Autodesk Inventor part; units mm, degrees
ref_plane "YZ Plane" through (0, 0, 0) normal (1, 0, 0) x (0, 1, 0)
ref_plane "XZ Plane" through (0, 0, 0) normal (0, 1, 0) x (-1, 0, 0)
ref_plane "XY Plane" through (0, 0, 0) normal (0, 0, 1) x (1, 0, 0)
sketch "Sketch1" plane through (0, 0, 0) normal (0, 1, 0) x (-1, 0, 0)
  line L0 (0, -471.17) -> (0, 471.17)
  line L1 (1409.065, 0) -> (-1409.065, 0)
  line L2 (-1003.3, 333.375) -> (1003.3, 333.375)
  line L3 (1003.3, 333.375) -> (1003.3, -333.375)
  line L4 (1003.3, -333.375) -> (-1003.3, -333.375)
  line L5 (-1003.3, -333.375) -> (-1003.3, 333.375)
  line L6 (-968.375, 298.45) -> (968.375, 298.45)
  line L7 (968.375, 298.45) -> (968.375, -298.45)
  line L8 (968.375, -298.45) -> (-968.375, -298.45)
  line L9 (-968.375, -298.45) -> (-968.375, 298.45)
  line L10 (-1006.475, 336.55) -> (1006.475, 336.55)
  line L11 (1006.475, 336.55) -> (1006.475, -336.55)
  line L12 (1006.475, -336.55) -> (-1006.475, -336.55)
  line L13 (-1006.475, -336.55) -> (-1006.475, 336.55)
  point P0 (0, 0)
  dimension "d0" = 2006.6
  dimension "d1" = 666.75
  dimension "d2" = 596.9
  dimension "d3" = 1936.75
  dimension "d4" = 3.175
  dimension "d5" = 3.175
extrude "Extrusion1" add sketch "Sketch1" against normal blind 3.175 contours L12 L13 L1 L5 L4 L0 | L0 L4 L3 L1 L11 L12 | L4 L5 L1 L9 L8 L0 | L0 L8 L7 L1 L3 L4 | L1 L3 L2 L0 L10 L11 | L13 L10 L0 L2 L5 L1 | L1 L7 L6 L0 L2 L3 | L5 L2 L0 L6 L9 L1
extrude "Extrusion2" add sketch "Sketch1" along normal blind 34.925 contours L12 L13 L1 L5 L4 L0 | L0 L4 L3 L1 L11 L12 | L1 L3 L2 L0 L10 L11 | L13 L10 L0 L2 L5 L1
sketch "Sketch2" plane through (0, 34.925, 0) normal (0, 1, 0) x (1, 0, 0)
  line L0 (1006.475, -336.55) -> (1006.475, 336.55)
  line L1 (1006.475, 336.55) -> (-1006.475, 336.55)
  line L2 (971.55, 336.55) -> (1006.475, 336.55)
  line L3 (1006.475, 339.725) -> (971.55, 339.725)
  line L4 (971.55, 339.725) -> (971.55, 336.55)
  line L5 (1006.475, 339.725) -> (1009.65, 339.725)
  line L6 (1009.65, 339.725) -> (1009.65, 301.625)
  line L7 (1009.65, 301.625) -> (1006.475, 301.625)
  line L8 (1006.475, 301.625) -> (1006.475, 336.55)
  point P0 (0, 0)
  dimension "d10" = 3.175
  dimension "d15" = 3.175
  dimension "d41" = 38.1
  dimension "d42" = 38.1
extrude "Extrusion3" add sketch "Sketch2" against normal blind 381
sketch "Sketch4" plane through (1006.475, -3.175, 336.55) normal (1, 0, 0) x (0, 0, -1)
  line L0 (638.175, 0) -> (0, 0)
  line L1 (447.479, 24.9105) -> (420.7746, -2.2646)
  line L2 (420.7746, -2.2646) -> (638.175, -215.9)
  line L3 (638.175, -215.9) -> (638.175, -162.483)
  line L4 (638.175, -162.483) -> (447.479, 24.9105)
  line L5 (638.175, 38.1) -> (638.175, -342.9)
  line L6 (676.275, -342.9) -> (638.175, -342.9)
  line L7 (422.9999, 0) -> (638.175, -211.4486)
  line L8 (422.9999, 0) -> (420.7746, -2.2646)
  line L9 (420.7746, -2.2646) -> (638.175, -215.9)
  line L10 (638.175, -215.9) -> (638.175, -211.4486)
  line L11 (638.175, -211.4486) -> (422.9999, 0)
  point P0 (336.55, 3.175)
  dimension "d23" = 38.1
  dimension "d24" = 304.8
  dimension "d25" = 127
  dimension "d28" = 3.175
extrude "Extrusion5" add sketch "Sketch4" against normal blind 34.925 contours L7 L3 L2 L1
extrude "Extrusion6" add sketch "Sketch4" along normal blind 3.175 contours L4 L3 L7 L0 | L0 L1 L4 | L7 L3 L2 L1
sketch "Sketch5" plane through (1009.65, 34.925, -339.725) normal (0, 0, -1) x (-1, 0, 0)
  line L0 (38.1, -381) -> (0, -381)
  line L1 (38.1, 0) -> (38.1, -381)
  line L2 (38.1, 0) -> (38.1, -38.1)
  line L3 (2016.125, -38.1) -> (38.1, -38.1)
  line L4 (2016.125, 0) -> (2016.125, -38.1)
  line L5 (38.1, 0) -> (2016.125, 0)
  line L6 (38.1, -355.6) -> (369.2808, -40.3999)
  line L7 (369.2808, -40.3999) -> (343.0141, -12.8015)
  line L8 (343.0141, -12.8015) -> (38.1, -303.0024)
  line L9 (38.1, -303.0024) -> (38.1, -355.6)
  line L10 (367.0919, -38.1) -> (38.1, -351.2169)
  point P0 (1009.65, -34.925)
  dimension "d33" = 38.1
  dimension "d34" = 25.4
  dimension "d35" = 3.175
  dimension "d36" = 457.2
extrude "Extrusion7" add sketch "Sketch5" against normal blind 3.175 contours L8 L3 L10 L1 | L8 L7 L3 | L10 L7 L6 L1
extrude "Extrusion8" add sketch "Sketch5" against normal blind 38.1 contours L10 L7 L6 L1
mirror "Mirror1" about plane through (0, 0, 0) normal (0, 0, 1) of "Extrusion8", "Extrusion7", "Extrusion6", "Extrusion5", "Extrusion3"
mirror "Mirror2" about plane through (0, 0, 0) normal (1, 0, 0) of "Extrusion8", "Extrusion7", "Extrusion6", "Extrusion5", "Extrusion3", "Mirror1"
properties part number "Burner_Stand"
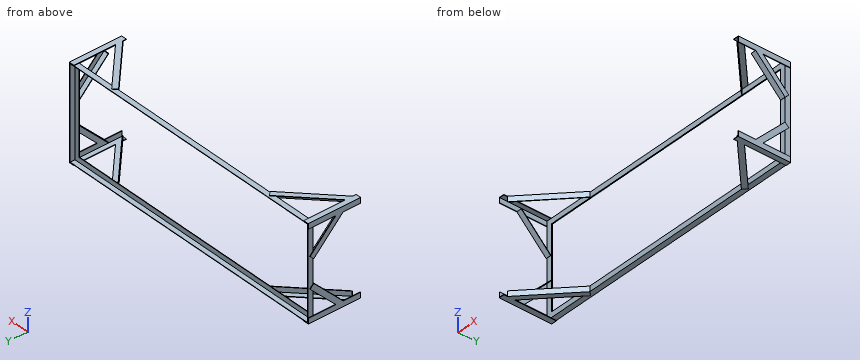
Can you work these out from the model? Positions are in its coordinate system, mm. Coordinates: 2 decimals unless noted, no trailing zeros. Loops run counter-clockwise (first coordinate to the right, second up) from the corner with the lowest first, then second, coordinate; pieces in that order, holes last. Notation, with made-up numbers: (-25.75, 29.25) - (-0.75, 29.25) arc R10 cw to (-0.75, 39.25) - close; hole circle Ø1 at (23.5, -33.75). An arc over 180 degrees is marked (long way). Use a Markdown table: item, result.
Item 1: I want a section at B-B on x = -89. Please give me the cut outline in (y, z) (3 decimals).
Numbers:
| item | result |
|---|---|
| outline | (-3.175, -336.55) - (34.925, -336.55) - (34.925, -333.375) - (0, -333.375) - (0, -298.45) - (-3.175, -298.45) - close; (-3.175, 298.45) - (0, 298.45) - (0, 333.375) - (34.925, 333.375) - (34.925, 336.55) - (-3.175, 336.55) - close |
Item 2: I want a section at D-D on x = -825.5. Please give me the cut outline in (y, z) (3 decimals).
Numbers:
| item | result |
|---|---|
| outline | (-181.672, -339.725) - (-129.075, -339.725) - (-129.075, -336.55) - (-177.289, -336.55) - (-177.289, -301.625) - (-181.672, -301.625) - close; (-181.672, 301.625) - (-177.289, 301.625) - (-177.289, 336.55) - (-129.075, 336.55) - (-129.075, 339.725) - (-181.672, 339.725) - close; (-3.175, -336.55) - (34.925, -336.55) - (34.925, -333.375) - (0, -333.375) - (0, -298.45) - (-3.175, -298.45) - close; (-3.175, 298.45) - (0, 298.45) - (0, 333.375) - (34.925, 333.375) - (34.925, 336.55) - (-3.175, 336.55) - close |
Item 3: I want a section at A-A on z = -66.5. Please give me the cut outline in (x, y) (3 decimals), and give its area (3 significant figures).
Numbers:
| item | result |
|---|---|
| outline | (-1006.475, -3.175) - (-968.375, -3.175) - (-968.375, 0) - (-1003.3, 0) - (-1003.3, 34.925) - (-1006.475, 34.925) - close; (968.375, -3.175) - (1006.475, -3.175) - (1006.475, 34.925) - (1003.3, 34.925) - (1003.3, 0) - (968.375, 0) - close |
| area | 464 mm2 |
Item 4: If I drill on probe 1 along X at (y, z) = (-55, -157.5) (3 decimals); probe 2 along X at (y, z) = (16, 297) (3 decimals); probe 3 along Y at (x, z) = (-226, -311) (3 decimals), over which ranges is the centre line in solid material (lowest first)? Write a range as from..to.
Numbers:
| item | result |
|---|---|
| probe 1 | x = -1009.65..-1006.475, 1006.475..1009.65 |
| probe 2 | x = -1006.475..-1003.3, 1003.3..1006.475 |
| probe 3 | y = -3.175..0 |
Item 5: I want a section at C-C on z = -250. Please give me the cut outline in (x, y) (3 decimals), and give its area (3 significant figures).
Numbers:
| item | result |
|---|---|
| outline | (-1009.65, -168.344) - (-971.55, -168.344) - (-971.55, -163.893) - (-1006.475, -163.893) - (-1006.475, -114.927) - (-1009.65, -114.927) - close; (-1006.475, -3.175) - (-968.375, -3.175) - (-968.375, 0) - (-1003.3, 0) - (-1003.3, 34.925) - (-1006.475, 34.925) - close; (968.375, -3.175) - (1006.475, -3.175) - (1006.475, 34.925) - (1003.3, 34.925) - (1003.3, 0) - (968.375, 0) - close; (971.55, -168.344) - (1009.65, -168.344) - (1009.65, -114.927) - (1006.475, -114.927) - (1006.475, -163.893) - (971.55, -163.893) - close |
| area | 1,110 mm2 |
